from build123d import *

# Parameters (mm, degrees)
SKETCH1_R           = 6
BOSS_EXTRUDE1_DEPTH = 30
SKETCH2_R           = 1.65
CUT_EXTRUDE1_DEPTH  = 41.902322672
CUT_EXTRUDE2_DEPTH  = 37.193922142


with BuildPart() as part:
    # Sketch1 → Boss-Extrude1 (new body)
    with BuildSketch(Plane(origin=(0, 0, 0), x_dir=(1, 0, 0), z_dir=(0, 1, 0))):
        Polygon((17, 11), (17, 5), (14.998887809, 2.998887809), (14.998887809, -7.001112191), (8.998887809, -7.001112191), (5, -11), (-5, -11), (-8.998887809, -7.001112191), (-14.998887809, -7.001112191), (-14.998887809, 2.998887809), (-17, 5), (-17, 11), align=None)
        with Locations(Location((0, 0, 0), (0, 0, 270))):
            Circle(SKETCH1_R, mode=Mode.SUBTRACT)
    extrude(amount=BOSS_EXTRUDE1_DEPTH)

    # Sketch2 → Cut-Extrude1 (cut, through all)
    with BuildSketch(Plane(origin=(0, 0, -11), x_dir=(-1, 0, 0), z_dir=(0, 0, -1))):
        with Locations((12, 6)):
            Circle(SKETCH2_R)
        with Locations(Location((-12, 6, 0), (0, 0, 180))):
            Circle(SKETCH2_R)
        with Locations((12, 24)):
            Circle(SKETCH2_R)
        with Locations((-12, 24)):
            Circle(SKETCH2_R)
    extrude(amount=-CUT_EXTRUDE1_DEPTH, mode=Mode.SUBTRACT)

    # Sketch3 → Cut-Extrude2 (cut, through all)
    with BuildSketch(Plane.XZ):
        Polygon((-6.31588303, -10.31588303), (6.31588303, -10.31588303), (7, -11), (-7, -11), align=None)
    extrude(amount=-CUT_EXTRUDE2_DEPTH, mode=Mode.SUBTRACT)


solid = part.part
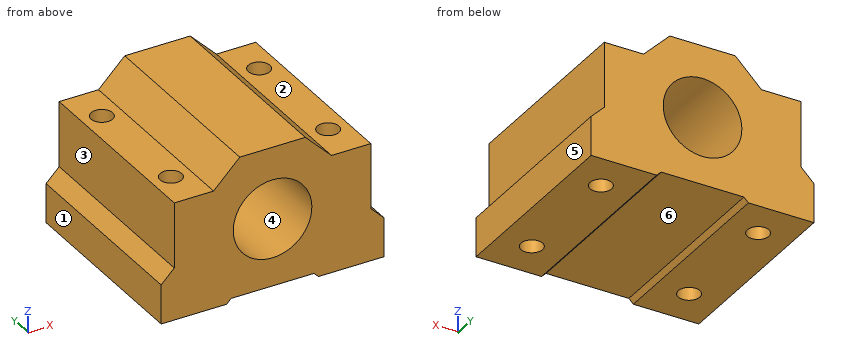
Can you work these out from the model? Positions are in its coordinate system, mm. Face numbers are marked on the shaded views. A direction names the side the tool comes from. Give positions to 0.01 mm unless a question says otherwise; leave off trailing zeros. Loops run counter-clockwise (first coordinate to the right, second up) from the corner with the lowest first, then second, coordinate; pieces in that order, holes last. Notation, with made-up numbers: M 39.5,48.25 L 61.5,48.25 A9 ccw 61.5,52.25 Z; hole C 60,68 d10. An arc over 180 degrees is marked long. One line per item, written item: value.
1) Imagine slicing it at C-C on y = 6. Write out the boundary of the cut face in (x, z).
Geometry check:
outline: M -17,-11 L -13.65,-11 L -13.65,7 L -15,7 L -15,-3 L -17,-5 Z; M -10.35,-11 L -7,-11 L -6.32,-10.32 L 6.32,-10.32 L 7,-11 L 10.35,-11 L 10.35,7 L 9,7 L 5,11 L -5,11 L -9,7 L -10.35,7 Z; M 13.65,-11 L 17,-11 L 17,-5 L 15,-3 L 15,7 L 13.65,7 Z; hole C 0,0 d12
2) Please list where these lines run through material, in increasing order: line 1 (Y direction, x = -12, z = -5); line 2 (Z direction, x = -9, y = 16.5); line 3 (X direction, y = 26.5, z = 5.5).
Geometry check:
line 1: y = 0 to 4.35, 7.65 to 22.35, 25.65 to 30
line 2: z = -11 to 7
line 3: x = -15 to -2.4, 2.4 to 15
3) Imagine slicing it at B-B on z = 0. Write out the boundary of the cut face in (x, y), and give its area (3 significant figures).
Geometry check:
outline: M -15,0 L -6,0 L -6,30 L -15,30 Z; M 6,0 L 15,0 L 15,30 L 6,30 Z; hole C -12,6 d3.3; hole C -12,24 d3.3; hole C 12,6 d3.3; hole C 12,24 d3.3
area: 506 mm²
4) On a 3-axis mill with a long thin cutter (end or side, diameter ignored), from which of +Z, -Z, +X, -X, +Y, -Y can I reach the whole of each face in a straight line? I mean the marked faces 1, 2 and 3. Say none if no direction works.
Geometry check:
face 1: +Z, -Z, -X, +Y, -Y
face 2: +Z, +X, +Y, -Y
face 3: +Z, -X, +Y, -Y
5) Imagine slicing it at A-A on x = 12. Write out the boundary of the cut face in (y, z).
Geometry check:
outline: M 0,-11 L 4.35,-11 L 4.35,7 L 0,7 Z; M 7.65,-11 L 22.35,-11 L 22.35,7 L 7.65,7 Z; M 25.65,-11 L 30,-11 L 30,7 L 25.65,7 Z
6) I'm going to push flat-ended pins straight in: pin 1 (10 mm diameter, centred on y = 17, z = -4.5, fed in from +X); pin 2 (3 mm diameter, centred on y = 14.5, z = 2, fed in from +X); pin 3 (2 mm diameter, centred on y = 23, z = 1, fed in from -X); pin 4 (5.5 mm diameter, centred on x = -12, y = 24, fed in from +Z). Where does each tip first touch, or does it pass through?
Geometry check:
pin 1: stops at x = 17
pin 2: stops at x = 15
pin 3: stops at x = -15
pin 4: stops at z = 7
7) Imagine slicing it at D-D on z = -7.75. Write out the boundary of the cut face in (x, y), and give its area (3 significant figures).
Geometry check:
outline: M -17,0 L 17,0 L 17,30 L -17,30 Z; hole C -12,6 d3.3; hole C -12,24 d3.3; hole C 12,6 d3.3; hole C 12,24 d3.3
area: 986 mm²
8) Thinking about a two-plate mould opening in Z: for the marked faces 4, 5 and 6, which applies, +Z half, -Z half, draft (parallel to the pull), parting line (faces both ways), or undercut?
Geometry check:
face 4: undercut
face 5: draft
face 6: -Z half
